Study the drawing (mm; zero at the part's minimum x, y, z) and answer. Round coordinates to 2 decimals unless told otherwise and drop trailing zeros. Write each loop counter-clockwise with the first axis right and the second up, starting at its lowest first coordinate (ties: lowest second). Pieces come first, ordered by that corner, then holes. Notation, with made-up numbers: (16, 0) - (37, 0) arc R23 ccw to (37, 11) - close; hole circle Ø10 at (70, 26.25). An arc over 180 degrees is marked (long way). Return JSON: item names as keys, results as strings. Group by question number.
(1) Section B-B, the plane y = 33.75 is taken. Write down the section's boundary in (x, z).
(2) Find the intervals of material crossed by line 1 along Y through (x, z) = (130, 1.2); line 2 along Y through (x, z) = (57, 1.2); line 3 along Y through (x, z) = (34, 1.25), in increasing order. Write a range as [from, to].
(3) Section A-A, the plane z = 3.4 is taken. Write down the section's boundary in (x, y) (3 decimals).
(4) Each of these flat-tipped pins is pushed along its axis until it touches: pin 1 (1.5 mm diameter, centred on x = 97, z = 2, fed in from -Y); pin 2 (1 mm diameter, centred on x = 34, z = 2.5, fed in from -Y); pin 3 (1.5 mm diameter, centred on y = 8.5, z = 5, fed in from -X). Where does it stop, or does it pass through?
(5) Section C-C, the plane y = 11.25 is taken. Write down the section's boundary in (x, z), then the cut area to 3 significant figures.
(6) Section D-D, the plane y = 5 is taken. Write down the section's boundary in (x, z), then the cut area to 3 significant figures.
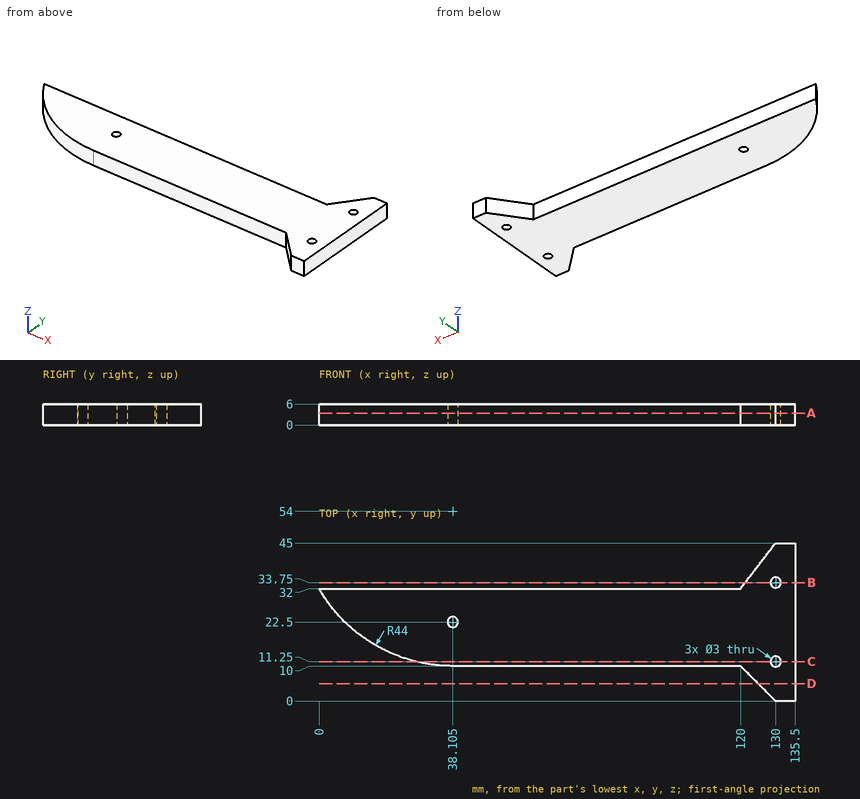
Working result:
{
 "1": {"outline": "(121.35, 0) - (128.5, 0) - (128.5, 6) - (121.35, 6) - close; (131.5, 0) - (135.5, 0) - (135.5, 6) - (131.5, 6) - close"},
 "2": {"line 1": "y = [0, 9.75], [12.75, 32.25], [35.25, 45]", "line 2": "y = [10, 32]", "line 3": "y = [10.19, 32]"},
 "3": {"outline": "(0, 32) arc R44 ccw to (38.105, 10) - (120, 10) - (130, 0) - (135.5, 0) - (135.5, 45) - (130, 45) - (120, 32) - close; hole circle Ø3 at (38.105, 22.5); hole circle Ø3 at (130, 11.25); hole circle Ø3 at (130, 33.75)"},
 "4": {"pin 1": "stops at y = 10", "pin 2": "stops at y = 10.15", "pin 3": "stops at x = 120.75"},
 "5": {"outline": "(27.69, 0) - (128.5, 0) - (128.5, 6) - (27.69, 6) - close; (131.5, 0) - (135.5, 0) - (135.5, 6) - (131.5, 6) - close", "area": "629 mm^2"},
 "6": {"outline": "(125, 0) - (135.5, 0) - (135.5, 6) - (125, 6) - close", "area": "63.0 mm^2"}
}
